Can you work these out from the model? Positions are in its coordinate system, mm. Round coordinates to 2 decimals unless told otherwise and drop trailing zeros. Write each loop counter-clockwise with the first axis right and the second up, starting at its lowest first coordinate (ties: lowest second). Pieces come first, ordered by that corner, then holes. Notation, with made-up numbers: M 66,44.25 L 117,44.25 A14 cw 117,60.25 Z; hole C 5.5,82 d4. An arc over 180 degrees is marked long. Use one line per item in the form item = value. Start each with the question number.
```python
from build123d import *

# Parameters (mm, degrees)
SKETCH1_R           = 5
SKETCH1_W           = 40
SKETCH1_H           = 40
BOSS_EXTRUDE1_DEPTH = 4


with BuildPart() as part:
    # Sketch1 → Boss-Extrude1 (new body)
    # profile 1 of 2: a face of its own
    with BuildSketch(Plane(origin=(0, 0, 0), x_dir=(1, 0, 0), z_dir=(0, 1, 0))):
        with BuildLine():
            ThreePointArc((60, 40), (80, 20), (60, 0))
            Line((60, 0), (40, 0))
            Line((40, 0), (40, 40))
            Line((40, 40), (60, 40))
        make_face()
        with Locations(Location((60, 20, 0), (0, 0, 270))):
            Circle(SKETCH1_R, mode=Mode.SUBTRACT)
    # profile 2 of 2: a face of its own
    with BuildSketch(Plane(origin=(0, 0, 0), x_dir=(1, 0, 0), z_dir=(0, 1, 0))):
        with Locations((20, 20)):
            Rectangle(SKETCH1_W, SKETCH1_H)
    extrude(amount=BOSS_EXTRUDE1_DEPTH)


solid = part.part
```
1. Please list where these lines run through material, in increasing order: line 1 along X through (y, z) = (2.3, -20); line 2 along X through (y, z) = (1.95, -3); line 3 along X through (y, z) = (3.6, -27) (3 decimals).
2. Will these pins go through, and if not, where does the flat tip stop? pin 1 (1.5 mm diameter, centred on y = 3.5, z = -14, fed in from +X); pin 2 (13 mm diameter, centred on x = 60, z = -20, fed in from -Y).
3. If we section it at B-B (x = 56): List the corners of the cut face in (y, z) for me, and give its area (3 significant figures).
4. If we section it at A-A (z = -20): List the corners of the cut face in (x, y) for me.
5. If we section it at D-D (z = -32): List the corners of the cut face in (x, y) for me.
6. If we mould it in two halves opening along X, with no side actions, what happens to faces 1 (the face through (80, 2, -20)), 2 (the face through (39, 0, -20)), 3 (the face through (64.957, 1.972, -20.651)), 4 (the face through (0, 2, -20))? For each: pulls with the +X half, pulls with the -X half, needs draft (parallel to the pull), parting line crosses it, or undercut.
7. If we section it at C-C (y = 1.15): List the corners of the cut face in (x, z) for me, and give its area (3 significant figures).
Model answer:
q1.line_1 = 0 to 55, 65 to 80
q1.line_2 = 0 to 70.54
q1.line_3 = 0 to 78.735
q2.pin_1 = 79.3
q2.pin_2 = 0
q3.outline = M 0,-40 L 4,-40 L 4,-23 L 0,-23 Z; M 0,-17 L 4,-17 L 4,0 L 0,0 Z
q3.area = 136 mm2
q4.outline = M 0,0 L 55,0 L 55,4 L 0,4 Z; M 65,0 L 80,0 L 80,4 L 65,4 Z
q5.outline = M 0,0 L 76,0 L 76,4 L 0,4 Z
q6.face_1 = pulls with the +X half
q6.face_2 = needs draft
q6.face_3 = undercut
q6.face_4 = pulls with the -X half
q7.outline = M 0,-40 L 60,-40 A20 ccw 60,0 L 0,0 Z; hole C 60,-20 d10
q7.area = 2,950 mm2
